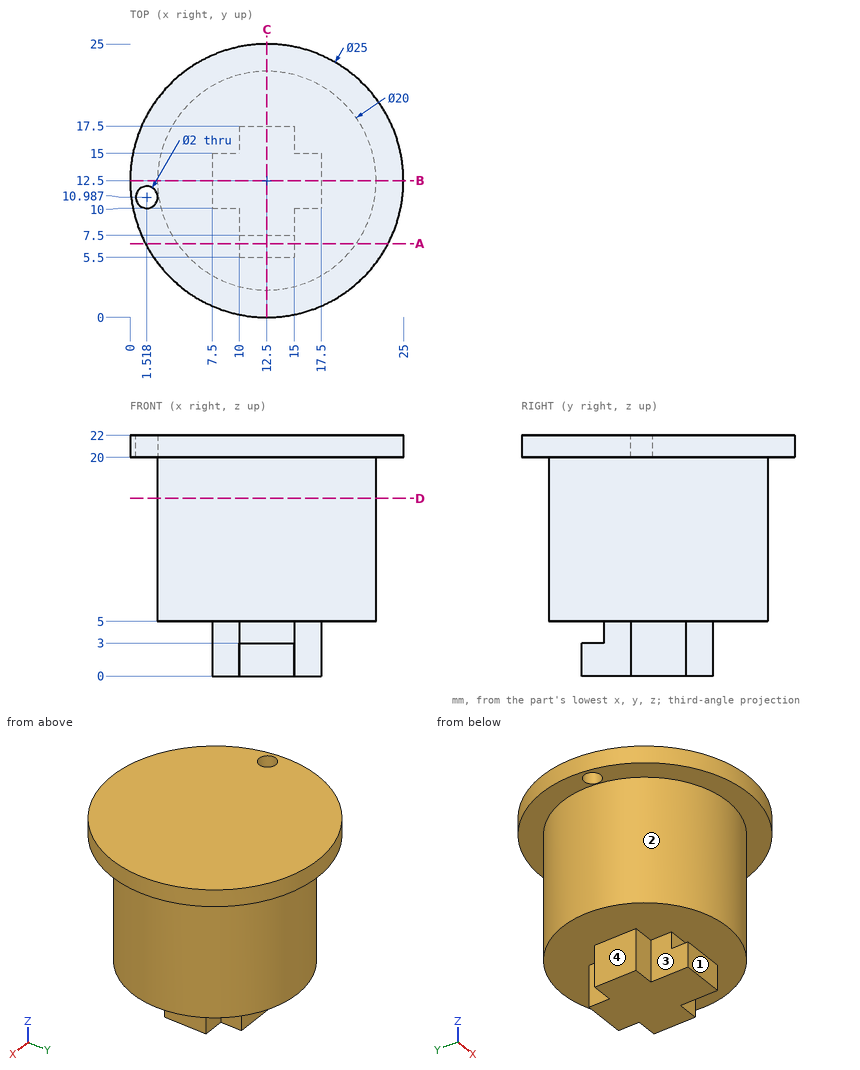
Part print with two shaded views. Sizes in mm from the minimum x, y, z corner. A direction names the side the tool comes from. Give positions to 0.01 mm unless a question says otherwise; leave off trailing zeros. Order: outer loops, then holes, each group sorted by start corner. A loop starts at its lowest first (then second) coordinate and runs counter-clockwise, first axis right, second up.
(1) Tool access for the marked faces 1, 2, 3 and 4: list every direction of +Z, -Z, +X, -X, +Y, -Y with a clear straight run to the whole face (end or side of a thin tool).
(2) Drill centre lines: L1, parallel to Y at x = 9, z = 2.75; L2, parallel to Z at x = 3.5, y = 14.5; L3, parallel to Y at x = 8.75, z = 14.5. Where is each one in solid material? Low to high.
(3) Flat gauge pins, fed straight in: pin 1 (0.8 mm diameter, centred on x = 16.5, z = 3, fed in from -Y); pin 2 (1.5 mm diameter, centred on x = 4, z = 9.5, fed in from -Y); pin 3 (1.5 mm diameter, centred on x = 13.5, z = 2.5, fed in from +Y). Where does each tip first touch, or does it go through?
(4) Saw through at D-D, the plane z = 16.25. Give the cut face in (x, y).
(5) Saw through at A-A, the plane y = 6.75. Give the cut face in (x, z).
(6) Saw through at C-C, the plane x = 12.5. Give the cut face in (y, z), then the cut area to 3 significant figures.
(7) Saw through at B-B, the plane y = 12.5. Give the cut face in (x, z), then the cut area to 3 significant figures.
Results found:
1. face 1: -Z, +X, -X, -Y
1. face 2: -Z
1. face 3: -Z, -X, -Y
1. face 4: -Z, -X, +Y, -Y
2. L1: y = 10 to 15
2. L2: z = 5 to 22
2. L3: y = 3.23 to 21.77
3. pin 1: stops at y = 10
3. pin 2: stops at y = 6.18
3. pin 3: stops at y = 17.5
4. outline: circle Ø20 at (12.5, 12.5)
5. outline: (1.4, 20) - (4.32, 20) - (4.32, 5) - (20.68, 5) - (20.68, 20) - (23.6, 20) - (23.6, 22) - (1.4, 22) - close; (10, 0) - (15, 0) - (15, 3) - (10, 3) - close
6. outline: (0, 20) - (2.5, 20) - (2.5, 5) - (7.5, 5) - (7.5, 3) - (5.5, 3) - (5.5, 0) - (17.5, 0) - (17.5, 5) - (22.5, 5) - (22.5, 20) - (25, 20) - (25, 22) - (0, 22) - close
6. area: 406 mm2
7. outline: (0, 20) - (2.5, 20) - (2.5, 5) - (7.5, 5) - (7.5, 0) - (17.5, 0) - (17.5, 5) - (22.5, 5) - (22.5, 20) - (25, 20) - (25, 22) - (0, 22) - close
7. area: 400 mm2
